```python
from build123d import *

# Parameters (mm, degrees)
SKETCH1_W                        = 41.73
SKETCH1_H                        = 30
BOSS_EXTRUDE1_DEPTH              = 5
SKETCH2_W                        = 10
SKETCH2_H                        = 20
BOSS_EXTRUDE3_DEPTH              = 144.78
BOSS_EXTRUDE5_DEPTH              = 1
BOSS_EXTRUDE5_DEPTH_BACK         = 8
SKETCH3_R                        = 27
SKETCH3_R_2                      = 22.5
SKETCH4_R                        = 22.5
CUT_EXTRUDE3_DEPTH               = 176.676886357
SKETCH7_R                        = 27
BOSS_EXTRUDE6_DEPTH              = 20
CUT_EXTRUDE5_START               = -18
SKETCH4_2_R                      = 22.5
CUT_EXTRUDE5_DEPTH               = 18
F_3_0MM_DOWEL_HOLE3_D            = 3
F_3_0MM_DOWEL_HOLE3_DEPTH        = 5
F_3_0MM_DOWEL_HOLE3_CSINK_D      = 3.05
F_3_0MM_DOWEL_HOLE3_CSINK_ANGLE  = 90
F_10_0MM_DOWEL_HOLE1_D           = 10
F_10_0MM_DOWEL_HOLE1_CSINK_D     = 10.05
F_10_0MM_DOWEL_HOLE1_CSINK_ANGLE = 90
F_3_0MM_DOWEL_HOLE4_D            = 3.2


with BuildPart() as part:
    # Sketch1 → Boss-Extrude1 (new body)
    with BuildSketch(Plane.XY):
        Rectangle(SKETCH1_W, SKETCH1_H)
    extrude(amount=BOSS_EXTRUDE1_DEPTH)

    # Sketch2 → Boss-Extrude3 (add)
    with BuildSketch(Plane(origin=(0, 0, 0), x_dir=(-1, 0, 0), z_dir=(0, 0, -1))):
        Rectangle(SKETCH2_W, SKETCH2_H)
    extrude(amount=BOSS_EXTRUDE3_DEPTH)

    # Sketch3 → Boss-Extrude5 (add, two sides: drawn at the far end of the back side and taken through both)
    with BuildSketch(Plane(origin=(0, 10, 0), x_dir=(1, 0, 0), z_dir=(0, 1, 0)).offset(-BOSS_EXTRUDE5_DEPTH_BACK)):
        with Locations(Location((0, 144.78, 0), (0, 0, 270))):
            Circle(SKETCH3_R)
        with Locations(Location((0, 144.78, 0), (0, 0, 270))):
            Circle(SKETCH3_R_2, mode=Mode.SUBTRACT)
    extrude(amount=BOSS_EXTRUDE5_DEPTH + BOSS_EXTRUDE5_DEPTH_BACK)

    # Sketch4 → Cut-Extrude3 (cut, through all)
    with BuildSketch(Plane(origin=(0, 10, 0), x_dir=(1, 0, 0), z_dir=(0, 1, 0))):
        with Locations(Location((0, 144.78, 0), (0, 0, 270))):
            Circle(SKETCH4_R)
    extrude(amount=-CUT_EXTRUDE3_DEPTH, mode=Mode.SUBTRACT)

    # Sketch7 → Boss-Extrude6 (add)
    with BuildSketch(Plane(origin=(0, 10, 0), x_dir=(1, 0, 0), z_dir=(0, 1, 0))):
        with Locations(Location((0, 144.78, 0), (0, 0, 270))):
            Circle(SKETCH7_R)
    extrude(amount=-BOSS_EXTRUDE6_DEPTH)

    # Sketch4<2> → Cut-Extrude5 (cut)
    with BuildSketch(Plane(origin=(0, 10, 0), x_dir=(1, 0, 0), z_dir=(0, 1, 0)).offset(CUT_EXTRUDE5_START)):
        with Locations(Location((0, 144.78, 0), (0, 0, 270))):
            Circle(SKETCH4_2_R)
    extrude(amount=CUT_EXTRUDE5_DEPTH, mode=Mode.SUBTRACT)

    # Ø3.0mm Dowel Hole3
    with Locations(Plane(origin=(0, 0, 0), x_dir=(-1, 0, 0), z_dir=(0, 0, -1))):
        with Locations((15, 8), (-15, 8), (15, -5), (-15, -5)):
            CounterSinkHole(F_3_0MM_DOWEL_HOLE3_D / 2, F_3_0MM_DOWEL_HOLE3_CSINK_D / 2, depth=F_3_0MM_DOWEL_HOLE3_DEPTH, counter_sink_angle=F_3_0MM_DOWEL_HOLE3_CSINK_ANGLE)

    # Ø10.0mm Dowel Hole1 (through all)
    with Locations(Plane(origin=(0, -8, 0), x_dir=(1, 0, 0), z_dir=(0, 1, 0))):
        with Locations((0, 144.78)):
            CounterSinkHole(F_10_0MM_DOWEL_HOLE1_D / 2, F_10_0MM_DOWEL_HOLE1_CSINK_D / 2, counter_sink_angle=F_10_0MM_DOWEL_HOLE1_CSINK_ANGLE)

    # Ø3.0mm Dowel Hole4 (through all)
    with Locations(Plane(origin=(0, -8, 0), x_dir=(1, 0, 0), z_dir=(0, 1, 0))):
        with Locations((0, 128.78), (0, 136.78), (16, 144.78), (9.5, 144.78), (0, 160.78), (0, 152.78), (-16, 144.78), (-9.5, 144.78)):
            Hole(F_3_0MM_DOWEL_HOLE4_D / 2)


solid = part.part
```
Check sheet for the modelled part. Datum: model origin and axes. Units: mm. A direction names the side the tool comes from. Round coordinates to 2 decimals unless told otherwise and drop trailing zeros. Write each loop counter-clockwise with the first axis right and the second up, starting at its lowest first coordinate (ties: lowest second). Pieces come first, ordered by that corner, then holes. Notation, with made-up numbers: (40, 80.25) -> (56, 80.25) arc R23 ccw to (56, 110.25) -> close; hole circle Ø3 at (73, 70.5). An arc over 180 degrees is marked (long way). One line per question, with ' | ' between items. Start each with the question number.
1. Sectioned sample at B-B, the plane z = -128.78. Record the cut outline in (x, y).
2. Depth check by flat-ended pin: pin 1 (5 mm diameter, centred on x = -9.5, z = -144.78, fed in from -Y); pin 2 (1.5 mm diameter, centred on x = 5, y = 6, fed in from -Z); pin 3 (6 mm diameter, centred on y = -0.5, z = -58, fed in from +X); pin 4 (8 mm diameter, centred on x = 10.5, z = -97.5, fed in from +Y). Enter the tip coordinate at first touch or a pass-through.
3. Scan lines: line 1 along Y through (x, z) = (15, 3.1); line 2 along X through (y, z) = (-9.15, -144.78); line 3 along X through (y, z) = (8, 2.05) (3 decimals). Record each from-to range of solid material in increasing order. Write a range as from..to.
4. Sectioned sample at A-A, the plane y = 8. Record the cut outline in (x, z) (3 decimals).
5. Set-up check for faces 4 (the face through (13.8, 7.1, 2.5)), 5 (the face through (-8.618, 1.633, -123.996)), 6 (the face through (0, -15, 2)), 7 (the face through (0.208, -9.014, -162.366)), 8 (the face through (0, 10, -58)): record each of +Z, -Z, +X, -X, +Y, -Y from which the full face is reachable in a straight line by a thin tool's end or side.
6. Release check for a two-part mould opening along Z. For faces 1 (the face through (0, 0, 5)), 2 (the face through (5, 0, -58)), 3 (the face through (0, -10, -117)) record: +Z half, -Z half, draft (parallel to the pull), parting line (faces both ways), or undercut.
7. Sectioned sample at C-C, the plane x = 0. Count the separate pieces of the cut face and the enclosed holes in it, then the cut area to 3 significant figures.
8. Sectioned sample at D-D, the plane z = -71. Record the cut outline in (x, y).
Taken from the geometry:
1) outline: (-21.75, -10) -> (-1.6, -10) -> (-1.6, -8) -> (-15.82, -8) -> (-15.82, 11) -> (-21.75, 11) -> close; (1.6, -10) -> (21.75, -10) -> (21.75, 11) -> (15.82, 11) -> (15.82, -8) -> (1.6, -8) -> close
2) pin 1: stops at y = -10 | pin 2: stops at z = -171.44 | pin 3: stops at x = 5 | pin 4: passes through
3) line 1: y = -15..-6.5, -3.5..6.5, 9.5..15 | line 2: x = -27..-17.6, -14.4..-11.1, -7.9..-5, 5..7.9, 11.1..14.4, 17.6..27 | line 3: x = -20.865..-16.5, -13.5..13.5, 16.5..20.865
4) outline: (-20.865, 0) -> (-16.525, 0) -> (-16.5, 0.025) -> (-16.5, 5) -> (-20.865, 5) -> close; (-13.5, 0.025) -> (-13.475, 0) -> (-5, 0) -> (-5, -118.247) arc R27 ccw (long way) to (5, -118.247) -> (5, 0) -> (13.475, 0) -> (13.5, 0.025) -> (13.5, 5) -> (-13.5, 5) -> close; (16.5, 0.025) -> (16.525, 0) -> (20.865, 0) -> (20.865, 5) -> (16.5, 5) -> close; hole circle Ø45 at (0, -144.78)
5) face 4: +Z | face 5: +Y | face 6: +Z, -Z, +X, -X, -Y | face 7: +Y, -Y | face 8: +X, -X, +Y
6) face 1: +Z half | face 2: undercut | face 3: draft
7) separate pieces: 6 | enclosed holes: 0 | area: 2,740 mm^2
8) outline: (-5, -10) -> (5, -10) -> (5, 10) -> (-5, 10) -> close
